The listing builds one solid part. Answer for the finished solid, in the listing's coordinates (mm). Coordinates: 2 decimals unless noted, no trailing zeros. Write each loop counter-clockwise with the first axis right and the second up, starting at its lowest first coordinate (ties: lowest second). Pieces come first, ordered by that corner, then holes.
(1) The part is cut by section C-C on y = -35.5. Determine the outline of the cut face in (x, z), plus the area to 3 significant figures.
(2) Given P1, Ø15, axis at x = 2004.5, y = -34.5, coming from the -Z side, flat-ended and moving along its own axis, determine where the tip first touches the part or whether it passes through.
(3) The part is cut by section B-B on z = 248. Determine the outline of the cut face in (x, y), plus the area to 3 significant figures.
(4) The part is cut by section D-D on x = 1866.5. Determine the outline of the cut face in (y, z), plus the area to 3 significant figures.
(5) The part is cut by section A-A on x = 2859. Determine the outline of the cut face in (y, z).
(6) Straight lines are drawn through the part: line 1 (X direction, y = -12.5, z = 411); line 2 (Z direction, x = 2600.5, y = -18); line 3 (X direction, y = -30.5, z = 693). For each, find the intervals that lie inside material, in ascending order.
from build123d import *

# Parameters (mm, degrees)
F0_W     = 1535
F0_H     = 1020
F0_W_2   = 700
F0_H_2   = 592.5
F0_H_3   = 930
F0_H_4   = 292.5
F1_DEPTH = 50
F2_W     = 15
F2_H     = 292.5
F3_DEPTH = 20


with BuildPart() as f1:
    # F0 (on Front) → F1 (new body)
    with BuildSketch(Plane.XZ):
        with Locations((767.5, 510)):
            Rectangle(F0_W, F0_H)
        with Locations((1140, 341.25)):
            Rectangle(F0_W_2, F0_H_2, mode=Mode.SUBTRACT)
        with Locations((395, 510)):
            Rectangle(F0_W_2, F0_H_3, mode=Mode.SUBTRACT)
        with Locations((1140, 828.75)):
            Rectangle(F0_W_2, F0_H_4, mode=Mode.SUBTRACT)
    extrude(amount=F1_DEPTH)

    # F2 (on Front) → F3 (join)
    with BuildSketch(Plane.XZ):
        Polygon((402.5, 975), (387.5, 975), (387.5, 675), (45, 675), (45, 660), (387.5, 660), (387.5, 360), (45, 360), (45, 345), (387.5, 345), (387.5, 45), (402.5, 45), (402.5, 345), (745, 345), (745, 360), (402.5, 360), (402.5, 660), (745, 660), (745, 675), (402.5, 675), align=None)
        Polygon((1132.5, 360), (790, 360), (790, 345), (1132.5, 345), (1132.5, 45), (1147.5, 45), (1147.5, 345), (1490, 345), (1490, 360), (1147.5, 360), (1147.5, 637.5), (1132.5, 637.5), align=None)
        with Locations((1140, 828.75)):
            Rectangle(F2_W, F2_H)
    extrude(amount=F3_DEPTH)


with BuildPart() as f4_1:
    # F4: instance of F1
    add(f1.part.mirror(Plane(origin=(1535, -25, 510), x_dir=(0, 1, 0), z_dir=(1, 0, 0))))


solid = f4_1.part
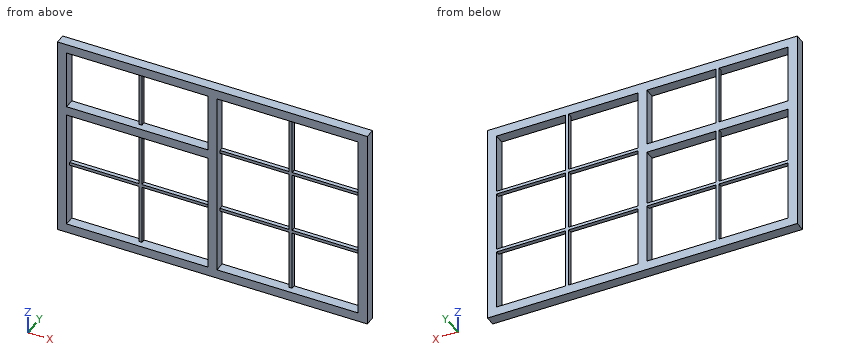
Model answer:
1. outline: (1535, 0) - (3070, 0) - (3070, 1020) - (1535, 1020) - close; hole (1580, 45) - (2280, 45) - (2280, 637.5) - (1580, 637.5) - close; hole (1580, 682.5) - (2280, 682.5) - (2280, 975) - (1580, 975) - close; hole (2325, 45) - (3025, 45) - (3025, 975) - (2325, 975) - close
1. area: 295,000 mm2
2. P1: stops at z = 0
3. outline: (1535, -50) - (1580, -50) - (1580, 0) - (1535, 0) - close; (1922.5, -20) - (1937.5, -20) - (1937.5, 0) - (1922.5, 0) - close; (2280, -50) - (2325, -50) - (2325, 0) - (2280, 0) - close; (2667.5, -20) - (2682.5, -20) - (2682.5, 0) - (2667.5, 0) - close; (3025, -50) - (3070, -50) - (3070, 0) - (3025, 0) - close
3. area: 7,350 mm2
4. outline: (-50, 0) - (0, 0) - (0, 45) - (-50, 45) - close; (-50, 637.5) - (0, 637.5) - (0, 682.5) - (-50, 682.5) - close; (-50, 975) - (0, 975) - (0, 1020) - (-50, 1020) - close; (-20, 345) - (0, 345) - (0, 360) - (-20, 360) - close
4. area: 7,050 mm2
5. outline: (-50, 0) - (0, 0) - (0, 45) - (-50, 45) - close; (-50, 975) - (0, 975) - (0, 1020) - (-50, 1020) - close; (-20, 345) - (0, 345) - (0, 360) - (-20, 360) - close; (-20, 660) - (0, 660) - (0, 675) - (-20, 675) - close
6. line 1: x = 1535 to 1580, 1922.5 to 1937.5, 2280 to 2325, 2667.5 to 2682.5, 3025 to 3070
6. line 2: z = 0 to 45, 345 to 360, 660 to 675, 975 to 1020
6. line 3: x = 1535 to 1580, 2280 to 2325, 3025 to 3070
